from build123d import *

# Parameters (mm, degrees)
F0_W      = 100
F0_H      = 100
F1_DEPTH  = 100
F3_R      = 12.5
F4_DEPTH  = 10
F7_R      = 12.5
F8_DEPTH  = 20
F10_R     = 12.5
F12_DEPTH = 10
F11_R     = 12.5
F13_DEPTH = 10
F14_R     = 12.5
F15_DEPTH = 10
F17_R     = 12.5
F18_DEPTH = 10
F19_R     = 11.5
F20_DEPTH = 10
F21_R     = 5


with BuildPart() as f1:
    # F0 (on Top) → F1 (new body)
    with BuildSketch(Plane.XY):
        Rectangle(F0_W, F0_H)
    extrude(amount=F1_DEPTH)

    # F3 (on face) → F4 (cut)
    with BuildSketch(Plane.XY.offset(100)):
        Circle(F3_R)
    extrude(amount=-F4_DEPTH, mode=Mode.SUBTRACT)

    # F7 (on face) → F8 (cut)
    with BuildSketch(Plane(origin=(-50, 0, 0), x_dir=(0, -1, 0), z_dir=(-1, 0, 0))):
        with Locations((-25, 50)):
            Circle(F7_R)
        with Locations((25, 50)):
            Circle(F7_R)
    extrude(amount=-F8_DEPTH, mode=Mode.SUBTRACT)

    # F10 (on face) → F12 (cut)
    with BuildSketch(Plane(origin=(0, 50, 0), x_dir=(-1, 0, 0), z_dir=(0, 1, 0))):
        with Locations((0, 50)):
            Circle(F10_R)
    extrude(amount=-F12_DEPTH, mode=Mode.SUBTRACT)

    # F11 (on face) → F13 (cut)
    with BuildSketch(Plane(origin=(0, 50, 0), x_dir=(-1, 0, 0), z_dir=(0, 1, 0))):
        with Locations((-25, 25)):
            Circle(F11_R)
        with Locations((25, 75)):
            Circle(F11_R)
    extrude(amount=-F13_DEPTH, mode=Mode.SUBTRACT)

    # F14 (on face) → F15 (cut)
    with BuildSketch(Plane.XZ.offset(50)):
        with Locations((-25, 75)):
            Circle(F14_R)
        with Locations((-25, 25)):
            Circle(F14_R)
        with Locations((25, 25)):
            Circle(F14_R)
        with Locations((25, 75)):
            Circle(F14_R)
    extrude(amount=-F15_DEPTH, mode=Mode.SUBTRACT)

    # F17 (on face) → F18 (cut)
    with BuildSketch(Plane.YZ.offset(50)):
        with Locations((-25, 75)):
            Circle(F17_R)
        with Locations((25, 75)):
            Circle(F17_R)
        with Locations((-25, 25)):
            Circle(F17_R)
        with Locations((25, 25)):
            Circle(F17_R)
        with Locations((0, 50)):
            Circle(F17_R)
    extrude(amount=-F18_DEPTH, mode=Mode.SUBTRACT)

    # F19 (on face) → F20 (cut)
    with BuildSketch(Plane(origin=(0, 0, 0), x_dir=(1, 0, 0), z_dir=(0, 0, -1))):
        with Locations((-25, 25)):
            Circle(F19_R)
        with Locations((-25, 0)):
            Circle(F19_R)
        with Locations((-25, -25)):
            Circle(F19_R)
        with Locations((25, -25)):
            Circle(F19_R)
        with Locations((25, 0)):
            Circle(F19_R)
        with Locations((25, 25)):
            Circle(F19_R)
    extrude(amount=-F20_DEPTH, mode=Mode.SUBTRACT)

    # F21
    f21_edges = [f1.edges().sort_by_distance(p)[0] for p in [
        (-50, 50, 50),
        (0, 50, 100),
        (50, 50, 50),
        (0, 50, 0),
        (50, 0, 0),
        (0, -50, 0),
        (-50, 0, 0),
        (-50, -50, 50),
        (50, -50, 50),
        (50, 0, 100),
        (0, -50, 100),
        (-50, 0, 100),
    ]]
    fillet(f21_edges, radius=F21_R)


solid = f1.part
Design review of the part built by this model. Coordinates are the model's own, in mm. A direction names the side the tool comes from. Round coordinates to 2 decimals unless told otherwise and drop trailing zeros. Loops run counter-clockwise (first coordinate to the right, second up) from the corner with the lowest first, then second, coordinate; pieces in that order, holes last. Notation, with made-up numbers: (14.25, 56) - (18.25, 56) arc R14 ccw to (18.25, 71) - close; hole circle Ø1 at (7, -40). An arc over 180 degrees is marked (long way). One line per question, with ' | ' between items.
1. Draft analysis for pull direction Z (two halves, no side actions). For faces 1 (the face through (0, 0, 90)), 2 (the face through (-14.03, -3.45, 4.93)), 3 (the face through (15.08, -45.07, 17.394)), state which applies: released by +Z, released by -Z, zero draft, split by the parting line, or undercut.
Results are:
face 1: released by +Z | face 2: zero draft | face 3: undercut
2. We need section C-C, the plane y = 0. State the section outline as (x, z) points.
Results are:
outline: (-50, 5) arc R5 ccw to (-45, 0) - (-36.5, 0) - (-36.5, 10) - (-13.5, 10) - (-13.5, 0) - (13.5, 0) - (13.5, 10) - (36.5, 10) - (36.5, 0) - (45, 0) arc R5 ccw to (50, 5) - (50, 37.5) - (40, 37.5) - (40, 62.5) - (50, 62.5) - (50, 95) arc R5 ccw to (45, 100) - (12.5, 100) - (12.5, 90) - (-12.5, 90) - (-12.5, 100) - (-45, 100) arc R5 ccw to (-50, 95) - close
3. For faces 4 (the face through (45.07, -2.71, 37.797)), 5 (the face through (-18.82, -34.7, 4.93)), 6 (the face through (25, 40, 25)), 7 (the face through (9, 50, 39)), 8 (the face through (-25, -40, 75)), list the 3-axis set-ups (+Z, -Z, +X, -X, +Y, -Y) from which the entire face can be reached by the end or side of a thin tool; tool diameter is ignored.
Results are:
face 4: +X | face 5: -Z | face 6: +Y | face 7: +Z, -Z, +X, -X, +Y | face 8: -Y
4. Clearance check with flat-ended pins moving along their axes: P1, Ø7, axis at x = 19.5, y = -24.5, coming from the -Z side; P2, Ø20, axis at y = 25, z = 50, coming from the -X side; P3, Ø7.5, axis at y = 21, z = 70, coming from the +X side. State where each tip first meets the part, or that it passes through.
Results are:
P1: stops at z = 10 | P2: stops at x = -30 | P3: stops at x = 40
5. We need section A-A, the plane x = -41. State the section outline as (y, z) points.
Results are:
outline: (-50, 5) arc R5 ccw to (-45, 0) - (45, 0) arc R5 ccw to (50, 5) - (50, 95) arc R5 ccw to (45, 100) - (-45, 100) arc R5 ccw to (-50, 95) - close; hole circle Ø25 at (-25, 50); hole circle Ø25 at (25, 50)
6. For L1, parallel to X at y = 0, z = 8; L2, parallel to Z at x = 44.5, y = -25; L3, parallel to Y at x = -25, z = 7.5, list the stretches that pass through material, from the lowest coordinate up. Write a range as [from, to].
Results are:
L1: x = [-50, -36.5], [-13.5, 13.5], [36.5, 50] | L2: z = [0, 12.5], [37.5, 62.5], [87.5, 100] | L3: y = [-50, -36.5], [-13.5, -11.5], [11.5, 13.5], [36.5, 50]
7. We need section B-B, the plane z = 65. State the section outline as (x, y) points.
Results are:
outline: (-50, -45) arc R5 ccw to (-45, -50) - (-32.5, -50) - (-32.5, -40) - (-17.5, -40) - (-17.5, -50) - (17.5, -50) - (17.5, -40) - (32.5, -40) - (32.5, -50) - (45, -50) arc R5 ccw to (50, -45) - (50, -32.5) - (40, -32.5) - (40, -17.5) - (50, -17.5) - (50, 17.5) - (40, 17.5) - (40, 32.5) - (50, 32.5) - (50, 45) arc R5 ccw to (45, 50) - (-17.5, 50) - (-17.5, 40) - (-32.5, 40) - (-32.5, 50) - (-45, 50) arc R5 ccw to (-50, 45) - close
